Geometry: final body of the model. Coordinates: model frame, mm. A direction names the side the tool comes from. Coordinates: 2 decimals unless noted, no trailing zeros. Write each loop counter-clockwise with the first axis right and the second up, starting at its lowest first coordinate (ties: lowest second). Pieces come first, ordered by that corner, then holes. Notation, with made-up numbers: (-36, -15.5) - (-24, -15.5) arc R26 cw to (-24, 20.5) - close; hole circle Ø6 at (73, 51). An arc over 180 degrees is marked (long way). Answer as a JSON object with one key per item and string values. Group by question number.
Item 1: Mould query, pull axis Z, two halves, no side actions, for faces 1 (the flat face through (0.99, 54.01, -373.94)), 2 (the flat face through (2, 136, -259)). Classes: pulls with the +Z half, pulls with the -Z half, needs draft (parallel to the pull), parting line crosses it, or undercut.
Item 2: First-contact query: pin 1 Ø0.6 at (x, z) = (1.5, -221) entering from -Y; pin 2 Ø0.6 at (x, y) = (0.5, -19.5) entering from +Z. Flat tips, straight axial feed; report the tip coordinate or a pass-through.
Item 3: Line query: line 1 along Z through (x, y) = (1.4, 55.5); line 2 along Z through (x, y) = (0.15, 51); line 3 along Z through (x, y) = (0.6, -7.5). Output: solid intervals per line, ascending. Write a range as from..to.
Item 4: Section A-A on y = 44.5. Return loops of the section in (x, z), and give its area (3 significant figures).
Item 5: Set-up query: faces 3 (the flat face through (0, 136, -259)), 4 (the flat face through (0.99, 49.03, -108.22)). Return all of +Z, -Z, +X, -X, +Y, -Y with unobstructed straight access to the full face (end or side cutting, diameter ignored); none if empty.
```python
from build123d import *

# Parameters (mm, degrees)
BOSS_EXTRUDE1_DEPTH = 2


with BuildPart() as part:
    # Sketch1 → Boss-Extrude1 (new body)
    with BuildSketch(Plane(origin=(0, 0, 0), x_dir=(0, 0, -1), z_dir=(1, 0, 0))):
        with BuildLine():
            Line((0, 0), (0, 332))
            add(Edge.make_bspline(
                [(0, 332), (217.959962459, 314.031089263), (510, 192.7)],
                knots=[0, 0, 0, 1, 1, 1], degree=2))
            Line((510, 192.7), (510, 0))
            Line((510, 0), (510, -65.5))
            Line((510, -65.5), (405, -65.5))
            Line((405, -65.5), (405, 12.5))
            Line((405, 12.5), (342, 96.7))
            Line((342, 96.7), (132.5, 96.7))
            Line((132.5, 96.7), (83.246188613, 0))
            Line((83.246188613, 0), (0, 0))
        make_face()
    extrude(amount=BOSS_EXTRUDE1_DEPTH)


solid = part.part
```
Checks:
{
 "1": {"face 1": "undercut", "face 2": "needs draft"},
 "2": {"pin 1": "y = 96.7", "pin 2": "z = -405"},
 "3": {"line 1": "-510..-372.83, -111.51..0", "line 2": "-510..-376.19, -109.22..0", "line 3": "-510..-405"},
 "4": {"outline": "(0, -510) - (2, -510) - (2, -381.06) - (0, -381.06) - close; (0, -105.91) - (2, -105.91) - (2, 0) - (0, 0) - close", "area": "470 mm^2"},
 "5": {"face 3": "+Z, -Z, -X, +Y, -Y", "face 4": "+X, -X, -Y"}
}
